```python
from build123d import *

# Parameters (mm, degrees)
SKETCH1_W           = 80
SKETCH1_H           = 80
BOSS_EXTRUDE1_DEPTH = 2
SKETCH2_W           = 80
SKETCH2_H           = 80
SKETCH2_W_2         = 78
SKETCH2_H_2         = 78
BOSS_EXTRUDE2_DEPTH = 15
FILLET1_R           = 20
FILLET2_R           = 10
FILLET3_R           = 20
FILLET4_R           = 10
SKETCH3_R           = 1
BOSS_EXTRUDE3_DEPTH = 6
SKETCH4_W           = 10
SKETCH4_H           = 10
BOSS_EXTRUDE4_DEPTH = 5
SKETCH5_W           = 6
SKETCH5_H           = 20
BOSS_EXTRUDE5_DEPTH = 20
CUT_EXTRUDE1_DEPTH  = 23
SKETCH7_R           = 2
CUT_EXTRUDE2_DEPTH  = 23
SKETCH8_R           = 3.5
CUT_EXTRUDE3_DEPTH  = 3
SKETCH9_R           = 1
CUT_EXTRUDE4_DEPTH  = 18
SKETCH10_R          = 1.5
CUT_EXTRUDE5_DEPTH  = 18
SKETCH11_R          = 69.283397128
CUT_EXTRUDE6_DEPTH  = 37


with BuildPart() as part:
    # Sketch1 → Boss-Extrude1 (new body)
    with BuildSketch(Plane.XY):
        with Locations((40, 40)):
            Rectangle(SKETCH1_W, SKETCH1_H)
    extrude(amount=BOSS_EXTRUDE1_DEPTH)

    # Sketch2 → Boss-Extrude2 (add)
    with BuildSketch(Plane.XY.offset(2)):
        with Locations((40, 40)):
            Rectangle(SKETCH2_W, SKETCH2_H)
        with Locations((40, 40)):
            Rectangle(SKETCH2_W_2, SKETCH2_H_2, mode=Mode.SUBTRACT)
    extrude(amount=BOSS_EXTRUDE2_DEPTH)

    # Fillet1
    fillet1_edges = [part.edges().sort_by_distance(p)[0] for p in [
        (1, 79, 9.5),
        (1, 1, 9.5),
        (79, 1, 9.5),
        (79, 79, 9.5),
    ]]
    fillet(fillet1_edges, radius=FILLET1_R)

    # Fillet2
    fillet2_edges = [part.edges().sort_by_distance(p)[0] for p in [
        (40, 1, 2),
        (79, 40, 2),
        (40, 79, 2),
        (1, 40, 2),
        (6.857864376, 73.142135624, 2),
        (73.142135624, 73.142135624, 2),
        (6.857864376, 6.857864376, 2),
        (73.142135624, 6.857864376, 2),
    ]]
    fillet(fillet2_edges, radius=FILLET2_R)

    # Fillet3
    fillet3_edges = [part.edges().sort_by_distance(p)[0] for p in [
        (0, 80, 8.5),
        (80, 80, 8.5),
        (80, 0, 8.5),
        (0, 0, 8.5),
    ]]
    fillet(fillet3_edges, radius=FILLET3_R)

    # Fillet4
    fillet4_edges = [part.edges().sort_by_distance(p)[0] for p in [
        (80, 40, 0),
        (0, 40, 0),
        (40, 80, 0),
        (40, 0, 0),
        (5.857864376, 5.857864376, 0),
        (5.857864376, 74.142135624, 0),
        (74.142135624, 74.142135624, 0),
        (74.142135624, 5.857864376, 0),
    ]]
    fillet(fillet4_edges, radius=FILLET4_R)

    # Sketch3 → Boss-Extrude3 (add)
    with BuildSketch(Plane.XY.offset(17)):
        with BuildLine():
            Line((72.292824946, 5.37212195), (70.635028843, 4.105439789))
            Line((70.635028843, 4.105439789), (70.635028843, 7.564971157))
            ThreePointArc((70.635028843, 7.564971157), (71.162236636, 8.837763364), (72.435028843, 9.364971157))
            Line((72.435028843, 9.364971157), (76.003973901, 9.364971157))
            Line((76.003973901, 9.364971157), (72.292824946, 5.37212195))
        make_face()
        with Locations((72.435028843, 7.564971157)):
            Circle(SKETCH3_R, mode=Mode.SUBTRACT)
        with BuildLine():
            Line((9.364971157, 4.105439789), (9.364971157, 7.564971157))
            ThreePointArc((9.364971157, 7.564971157), (8.837763364, 8.837763364), (7.564971157, 9.364971157))
            Line((7.564971157, 9.364971157), (3.996026099, 9.364971157))
            Line((3.996026099, 9.364971157), (7.707175054, 5.37212195))
            Line((7.707175054, 5.37212195), (9.364971157, 4.105439789))
        make_face()
        with Locations((7.564971157, 7.564971157)):
            Circle(SKETCH3_R, mode=Mode.SUBTRACT)
        with BuildLine():
            Line((70.635028843, 75.894560211), (70.635028843, 72.435028843))
            ThreePointArc((70.635028843, 72.435028843), (71.162236636, 71.162236636), (72.435028843, 70.635028843))
            Line((72.435028843, 70.635028843), (76.003973901, 70.635028843))
            Line((76.003973901, 70.635028843), (72.292824946, 74.62787805))
            Line((72.292824946, 74.62787805), (70.635028843, 75.894560211))
        make_face()
        with Locations((72.435028843, 72.435028843)):
            Circle(SKETCH3_R, mode=Mode.SUBTRACT)
        with BuildLine():
            Line((7.707175054, 74.62787805), (9.364971157, 75.894560211))
            Line((9.364971157, 75.894560211), (9.364971157, 72.435028843))
            ThreePointArc((9.364971157, 72.435028843), (8.837763364, 71.162236636), (7.564971157, 70.635028843))
            Line((7.564971157, 70.635028843), (3.996026099, 70.635028843))
            Line((3.996026099, 70.635028843), (7.707175054, 74.62787805))
        make_face()
        with Locations((7.564971157, 72.435028843)):
            Circle(SKETCH3_R, mode=Mode.SUBTRACT)
    extrude(amount=-BOSS_EXTRUDE3_DEPTH)

    # Sketch4 → Boss-Extrude4 (add)
    with BuildSketch(Plane(origin=(0, 0, 0), x_dir=(-1, 0, 0), z_dir=(0, 0, -1))):
        with Locations((-35, 35)):
            Rectangle(SKETCH4_W, SKETCH4_H)
        with Locations((-35, 45)):
            Rectangle(SKETCH4_W, SKETCH4_H)
        with Locations((-45, 45)):
            Rectangle(SKETCH4_W, SKETCH4_H)
        with Locations((-45, 35)):
            Rectangle(SKETCH4_W, SKETCH4_H)
    extrude(amount=BOSS_EXTRUDE4_DEPTH)

    # Sketch5 → Boss-Extrude5 (add)
    with BuildSketch(Plane(origin=(0, 0, -5), x_dir=(-1, 0, 0), z_dir=(0, 0, -1))):
        with Locations((-33, 40)):
            Rectangle(SKETCH5_W, SKETCH5_H)
        with Locations((-47, 40)):
            Rectangle(SKETCH5_W, SKETCH5_H)
    extrude(amount=BOSS_EXTRUDE5_DEPTH)

    # Sketch6 → Cut-Extrude1 (cut)
    with BuildSketch(Plane.ZY.offset(-30)):
        with BuildLine():
            Line((-15, 30), (-19.756708154, 21.186247086))
            Line((-19.756708154, 21.186247086), (-29.168380108, 27.64799201))
            Line((-29.168380108, 27.64799201), (-29.168380108, 53.846153493))
            Line((-29.168380108, 53.846153493), (-15, 50))
            ThreePointArc((-15, 50), (-25, 40), (-15, 30))
        make_face()
    extrude(amount=-CUT_EXTRUDE1_DEPTH, mode=Mode.SUBTRACT)

    # Sketch7 → Cut-Extrude2 (cut)
    with BuildSketch(Plane.ZY.offset(-30)):
        with Locations((-15, 40)):
            Circle(SKETCH7_R)
    extrude(amount=-CUT_EXTRUDE2_DEPTH, mode=Mode.SUBTRACT)

    # Sketch8 → Cut-Extrude3 (cut)
    with BuildSketch(Plane.ZY.offset(-30)):
        with Locations((-15, 40)):
            Circle(SKETCH8_R)
    extrude(amount=-CUT_EXTRUDE3_DEPTH, mode=Mode.SUBTRACT)

    # Sketch9 → Cut-Extrude4 (cut)
    with BuildSketch(Plane(origin=(0, 0, -5), x_dir=(-1, 0, 0), z_dir=(0, 0, -1))):
        with Locations((-40, 45)):
            Circle(SKETCH9_R)
        with Locations((-40, 35)):
            Circle(SKETCH9_R)
    extrude(amount=-CUT_EXTRUDE4_DEPTH, mode=Mode.SUBTRACT)

    # Sketch10 → Cut-Extrude5 (cut)
    with BuildSketch(Plane(origin=(0, 0, -5), x_dir=(-1, 0, 0), z_dir=(0, 0, -1))):
        with Locations((-40, 40)):
            Circle(SKETCH10_R)
    extrude(amount=-CUT_EXTRUDE5_DEPTH, mode=Mode.SUBTRACT)

    # Sketch11 → Cut-Extrude6 (cut)
    with BuildSketch(Plane(origin=(0, 0, 0), x_dir=(-1, 0, 0), z_dir=(0, 0, -1))):
        with Locations((-39.654791549, 38.656536987)):
            Circle(SKETCH11_R)
    extrude(amount=-CUT_EXTRUDE6_DEPTH, mode=Mode.SUBTRACT)


solid = part.part
```
Design review of the part built by this model. Coordinates are the model's own, in mm. A direction names the side the tool comes from. Coordinates: 2 decimals unless noted, no trailing zeros. Loops run counter-clockwise (first coordinate to the right, second up) from the corner with the lowest first, then second, coordinate; pieces in that order, holes last. Notation, with made-up numbers: (58.5, -6.5) - (81.5, -6.5) arc R20 ccw to (81.5, 23.5) - close; hole circle Ø5 at (-7.5, 50.25). An arc over 180 degrees is marked (long way). Use CSV: the item, a comma, the result in double quotes. Start each with the question number.
1) Wall thickness on L1, parallel to Y at x = 40, z = -3; L2, parallel to X at y = 37.5, z = -10; L3, parallel to Y at x = 32.3, z = -15: over which ranges is each line inside the solid? List them lowest first. Write a range as from..to.
2) Consider section C-C on y = 35.5. Write out the cut boundary in (x, z), then the cut area to 3 significant figures.
3) Consider section D-D on z = -16.5. Write out the cut boundary in (x, y).
4) The part is to be moulded in two halves that separate along X. For faces 3 (the flat face through (42, 40, -5)), 4 (the cylindrical face through (39.46, 45.84, -2.54)), 5 (the cylindrical face through (31.48, 43.47, -15.46)), 6 (the flat face through (33, 38, -13)), say which applies: +X half, -X half, draft (parallel to the pull), parting line (faces both ways), or undercut.
5) Consider section A-A on z = -6.5. Write out the cut boundary in (x, y), then the cut area to 3 significant figures.
6) Tool access review of faces 1 (the flat face through (44, 39.9, -12.6)), 2 (the flat face through (40, 50, -4)): name each direction out of +Z, -Z, +X, -X, +Y, -Y from which nothing blocks a thin tool from reaching the whole face with its end or side.
7) Consider section B-B on x = 47.5. Write out the cut boundary in (y, z), then the cut area to 3 significant figures.
8) For pin 1 Ø4 at (x, y) = (40, 44.5) entering from -Z; pin 2 Ø3 at (x, z) = (38.5, -21) entering from +Y; pin 3 Ø6 at (x, y) = (34, 46.5) entering from -Z; pin 4 Ø5 at (y, z) = (40, -15) entering from -X, all flat-tipped, find the tip position at first contact; note any pin that passes through.
Geometry says:
1,L1,"30..34, 36..38.5, 41.5..44, 46..50"
1,L2,"30..36, 44..50"
1,L3,"30..36.5, 43.5..50"
2,outline,"(30, -23.93) - (36, -23.93) - (36, -5) - (39.13, -5) - (39.13, 0) - (30, 0) - close; (40.87, -5) - (44, -5) - (44, -23.93) - (50, -23.93) - (50, 0) - (40.87, 0) - close"
2,area,"319 mm^2"
3,outline,"(30, 30.11) - (36, 30.11) - (36, 38.68) - (33, 38.68) - (33, 36.84) - (30, 36.84) - close; (30, 43.16) - (33, 43.16) - (33, 41.32) - (36, 41.32) - (36, 49.89) - (30, 49.89) - close; (44, 30.11) - (50, 30.11) - (50, 38.68) - (44, 38.68) - close; (44, 41.32) - (50, 41.32) - (50, 49.89) - (44, 49.89) - close"
4,face 3,"undercut"
4,face 4,"undercut"
4,face 5,"draft"
4,face 6,"-X half"
5,outline,"(30, 30) - (36, 30) - (36, 50) - (30, 50) - close; (44, 30) - (50, 30) - (50, 50) - (44, 50) - close"
5,area,"240 mm^2"
6,face 1,"-Z, +Y, -Y"
6,face 2,"+Z, -Z, +X, -X, +Y"
7,outline,"(30, -15) arc R10 ccw to (50, -15) - (50, 0) - (30, 0) - close; hole circle Ø4 at (40, -15)"
7,area,"445 mm^2"
8,pin 1,"z = -5"
8,pin 2,"through"
8,pin 3,"z = -24.37"
8,pin 4,"x = 33"
